Autodesk Inventor part; units mm, degrees
ref_plane "YZ Plane" through (0, 0, 0) normal (1, 0, 0) x (0, 1, 0)
ref_plane "XZ Plane" through (0, 0, 0) normal (0, 1, 0) x (-1, 0, 0)
ref_plane "XY Plane" through (0, 0, 0) normal (0, 0, 1) x (1, 0, 0)
sketch "Náčrt1" plane through (0, 0, 0) normal (0, 0, 1) x (1, 0, 0)
  line L0 (-40, 0) -> (40, 0) construction
  line L1 (-40, -5) -> (40, -5)
  line L2 (40, 5) -> (-40, 5)
  arc A0 (-40, 5) -> (-40, -5) centre (-40, 0) ccw
  arc A1 (40, -5) -> (40, 5) centre (40, 0) ccw
  point P0 (0, 0)
  point P1 (45, 0)
  dimension "d0" = 45
  dimension "d1" = 5
extrude "Vysunutí1" add sketch "Náčrt1" along normal blind 0.5
sketch "Náčrt2" plane through (0, 0, 0) normal (0, 0, -1) x (-1, 0, 0)
  arc A0 (40, -5) -> (40, 5) centre (40, 0) ccw
  circle A1 centre (40, 0) radius 2
  point P0 (0, 0)
  dimension "d4" = 4
extrude "Vysunutí2" cut sketch "Náčrt2" against normal through all
pattern_linear "Obdélníkové pole1" count 9 spacing 10 along (1, 0, 0) of "Vysunutí2"
properties part number "1009"
The model under review builds one solid part; all positions refer to its coordinate system, in mm. Round coordinates to 2 decimals unless told otherwise and drop trailing zeros. Loops run counter-clockwise (first coordinate to the right, second up) from the corner with the lowest first, then second, coordinate; pieces in that order, holes last. Notation, with made-up numbers: M 47,-33.5 L 104,-33.5 A25 cw 104,-19.5 Z; hole C 54.5,-25 d9. An arc over 180 degrees is marked long. Answer as a JSON object with one key per item and string values.
(1) Take a section at A-A on x = 20. Give the boundary of the cut face in (y, z).
Resolved:
{"outline": "M -5,0 L -2,0 L -2,0.5 L -5,0.5 Z; M 2,0 L 5,0 L 5,0.5 L 2,0.5 Z"}
(2) Draft analysis for pull direction X (two halves, no side actions). For faces 1 (the cylindrical face through (11.6, -1.2, 0.2)), 2 (the flat face through (-1, 2, 0.5)), 3 (the cylindrical face through (45, 0.1, 0.2)), 4 (the cylindrical face through (-38.002, 0.088, 0.246)), state which applies: released by +X, released by -X, zero draft, split by the parting line, or undercut.
Resolved:
{"face 1": "undercut", "face 2": "zero draft", "face 3": "released by +X", "face 4": "undercut"}
(3) Take a section at D-D on y = -3.25. Give the boundary of the cut face in (x, z), and give its area (3 significant figures).
Resolved:
{"outline": "M -43.8,0 L 43.8,0 L 43.8,0.5 L -43.8,0.5 Z", "area": "43.8 mm²"}
(4) To check wall thickness, follow line 1 along Y through (x, z) = (30, 0.3); line 2 along X through (y, z) = (4, 0.1); line 3 along Y through (x, z) = (39, 0.4). State the ranges of each line that lie inside material, in increasing order.
Resolved:
{"line 1": "-5 to -2, 2 to 5", "line 2": "-43 to 43", "line 3": "-5 to -1.73, 1.73 to 5"}
(5) Take a section at B-B on z = 0.15. Count the separate pieces of the cut face and the enclosed holes in it, and give its area (3 significant figures).
Resolved:
{"separate pieces": "1", "enclosed holes": "9", "area": "765 mm²"}
